Autodesk Inventor part; units mm, degrees
ref_plane "YZ Plane" through (0, 0, 0) normal (1, 0, 0) x (0, 1, 0)
ref_plane "XZ Plane" through (0, 0, 0) normal (0, 1, 0) x (-1, 0, 0)
ref_plane "XY Plane" through (0, 0, 0) normal (0, 0, 1) x (1, 0, 0)
sketch "Sketch3" plane through (0, 0, 0) normal (0, 0, 1) x (1, 0, 0)
  line L0 (-80.5781, 0.8246) -> (-80.5781, 20.7988) construction
  circle A0 centre (-80.5781, 0.8246) radius 13.481
  line L1 (-53.7179, 12.5571) -> (-53.7179, -10.9927)
  arc A1 (-53.7179, -10.9927) -> (-51.5054, -12.9814) centre (-51.7179, -10.9927) ccw
  arc A2 (-51.5054, 14.5458) -> (-53.7179, 12.5571) centre (-51.7179, 12.5571) ccw
  line L2 (36.2229, -3.6088) -> (-51.5054, -12.9814)
  line L3 (38.0104, 3.1845) -> (38.0104, -1.6201)
  line L4 (-80.5781, 0.8246) -> (49.5525, 0.8246) construction
  circle A3 centre (49.6953, -3.8247) radius 5.6609
  line L5 (59.6953, 14.884) -> (59.6953, -12.7998) construction
  spline S0 degree 4 poles (77.9414, 11.0338) (75.5683, 12.9654) (71.7145, 13.0272) (66.8099, 13.9036) (60.7685, 14.7338) (56.2959, 15.3578) (51.7728, 15.9509) (47.2242, 16.5426) (42.6244, 17.1111) (37.9974, 17.6651) (33.3378, 18.1987) (28.6546, 18.7114) (23.9504, 19.2026) (19.2309, 19.6699) (14.5002, 20.1135) (9.7632, 20.5291) (5.025, 20.9191) (0.2903, 21.2792) (-4.4372, 21.6095) (-9.151, 21.9092) (-13.8524, 22.1766) (-18.5268, 22.4102) (-23.2002, 22.6105) (-27.8558, 22.7627) (-32.4748, 22.8704) (-37.0553, 22.9312) (-41.5904, 22.9454) (-46.0738, 22.9127) (-50.5027, 22.8323) (-54.8678, 22.7052) (-59.1755, 22.5324) (-63.394, 22.3084) (-67.5752, 22.0492) (-71.5451, 21.7209) (-75.7777, 21.4072) (-79.04, 20.9063) (-83.4863, 20.5541) (-87.0067, 20.037) (-90.7113, 19.5168) (-94.2172, 18.9459) (-97.6363, 18.3426) (-100.9342, 17.7015) (-104.1216, 17.0263) (-107.1909, 16.3187) (-110.1396, 15.5797) (-112.9656, 14.8117) (-115.6652, 14.0172) (-118.2357, 13.1965) (-120.6759, 12.3541) (-122.9817, 11.4895) (-125.1529, 10.6071) (-127.1857, 9.7065) (-129.0794, 8.7914) (-130.8324, 7.8633) (-132.4429, 6.923) (-133.9096, 5.9737) (-135.2322, 5.016) (-136.4083, 4.0508) (-137.4392, 3.0816) (-138.3215, 2.1025) (-139.0592, 1.1321) (-139.6407, 0.1249) (-140.106, -0.8362) (-140.3589, -2.0477) (-140.602, -2.598) (-140.1166, -5.4607) (-140.0539, -5.4622) (-139.4639, -6.7645) (-138.8842, -7.4979) (-138.1173, -8.3934) (-137.2199, -9.1877) (-136.1721, -9.9852) (-134.9893, -10.738) (-133.6669, -11.4655) (-132.2091, -12.1599) (-130.6156, -12.8245) (-128.8897, -13.4579) (-127.0312, -14.0591) (-125.0439, -14.6296) (-122.9287, -15.1678) (-120.6879, -15.6738) (-118.3241, -16.1476) (-115.8396, -16.5892) (-113.2366, -16.9984) (-110.5176, -17.3742) (-107.6861, -17.7183) (-104.7439, -18.0297) (-101.6943, -18.3095) (-98.5398, -18.5568) (-95.2843, -18.7732) (-91.9297, -18.9579) (-88.48, -19.1131) (-84.9381, -19.2376) (-81.3071, -19.3341) (-77.5906, -19.4015) (-73.7915, -19.4421) (-69.9139, -19.4561) (-65.961, -19.445) (-61.9362, -19.4102) (-57.8434, -19.3518) (-53.6861, -19.2727) (-49.4679, -19.1731) (-45.1932, -19.0538) (-40.8649, -18.9183) (-36.4879, -18.766) (-32.0649, -18.5992) (-27.598, -18.4192) (-23.0941, -18.227) (-18.5434, -18.0273) (-13.9382, -17.8076) (-9.3141, -17.5719) (-4.666, -17.3195) (-0.0002, -17.052) (4.6675, -16.7728) (9.3655, -16.4759) (14.0236, -16.1832) (19.545, -15.7815) (23.3079, -15.6072) (27.1098, -15.1781) (28.8959, -15.0599) knots 0 0 0 0 0 0.024672 0.034555 0.0445 0.054495 0.064543 0.074632 0.084755 0.094911 0.105094 0.115299 0.125521 0.135755 0.145995 0.156237 0.166475 0.176705 0.186921 0.197118 0.207299 0.217463 0.227605 0.23772 0.247796 0.257824 0.267798 0.277713 0.287563 0.297345 0.307053 0.31668 0.326224 0.335555 0.344908 0.354162 0.363308 0.372467 0.381393 0.390196 0.398872 0.407415 0.41582 0.424082 0.432193 0.44015 0.447945 0.455574 0.46303 0.470307 0.477401 0.484305 0.491015 0.497525 0.503831 0.509931 0.515822 0.521506 0.526986 0.53227 0.537373 0.542316 0.547131 0.552525 0.557529 0.562533 0.567581 0.57205 0.576988 0.582082 0.587354 0.592817 0.598478 0.604341 0.610406 0.616671 0.623133 0.629789 0.636632 0.643658 0.650861 0.658236 0.665777 0.673478 0.681333 0.689338 0.697486 0.705771 0.71419 0.722736 0.731403 0.740188 0.749084 0.758087 0.767192 0.776393 0.785687 0.795067 0.804529 0.814069 0.823682 0.833362 0.843106 0.852907 0.862763 0.872667 0.88262 0.892624 0.902675 0.912766 0.92289 0.933033 0.943191 0.953358 0.963531 0.973703 0.984092 1 1 1 1 1
  line L6 (7.5013, -16.4763) -> (50.2906, -13.6435) construction
  arc A4 (44.8353, -17.2546) -> (13.385, -19.3367) centre (31.5327, -54.8885) ccw construction
  line L7 (159.6953, -3.8066) -> (59.6953, -3.8066) construction
  line L8 (-51.5054, 14.5458) -> (36.2229, 5.1732)
  arc A5 (36.2229, -3.6088) -> (38.0104, -1.6201) centre (36.0104, -1.6201) ccw
  arc A6 (38.0104, 3.1845) -> (36.2229, 5.1732) centre (36.0104, 3.1845) ccw
  spline S1 degree 4 poles (78.1029, 11.0141) (76.6463, 11.2227) (73.9909, 10.5042) (70.2765, 8.6041) (66.0429, 5.3938) (62.3889, 1.8499) (60.314, -1.2467) (59.5572, -3.5763) (59.5773, -5.0793) knots 0 0 0 0 0 0.302475 0.43895 0.576633 0.708802 1 1 1 1 1
  spline S2 degree 4 poles (28.8959, -15.0599) (34.0984, -14.7105) (49.269, -14.182) (58.5645, -15.239) (59.5773, -5.0793) knots 0 0 0 0 0 1 1 1 1 1
  line L9 (28.8959, -15.0599) -> (34.0984, -14.7105) construction
  line L10 (34.0984, -14.7105) -> (49.269, -14.182) construction
  line L11 (49.269, -14.182) -> (58.5645, -15.239) construction
  line L12 (58.5645, -15.239) -> (59.5773, -5.0793) construction
  line L13 (-140.4646, -2.8394) -> (159.4818, -3.8173) construction
  line L14 (-132.0856, 0.6333) -> (-132.0856, -6.3667)
  line L15 (-132.0856, -6.3667) -> (-110.3816, -12.3574)
  line L16 (-110.3816, -12.3574) -> (-104.797, -12.3574)
  line L17 (-104.797, -12.3574) -> (-104.797, -18.0156)
  line L18 (-132.0856, 0.6333) -> (-110.3816, 10.553)
  line L19 (-110.3816, 10.553) -> (-104.1736, 10.553)
  line L20 (-104.1736, 10.553) -> (-104.1736, 17.0026)
  line L21 (38.0104, 0.8246) -> (38.0104, -14.6534)
  line L22 (38.0104, 0.8246) -> (38.0104, 17.6585)
  point P0 (0, 0)
  point P1 (17.6589, 23.5628)
  point P2 (75.883, 10.8572)
  point P3 (72.8647, 9.7686)
  point P4 (69.4179, 7.8149)
  point P5 (66.0452, 5.2617)
  point P6 (63.1887, 2.4463)
  point P7 (61.1228, -0.3317)
  point P8 (59.9357, -2.8689)
  point P9 (-160.0931, -3.8671)
  point P10 (28.8959, -15.0599)
  point P11 (69.5533, 13.4647)
  point P12 (65.1899, 14.1023)
  point P13 (60.7936, 14.7318)
  point P14 (56.3207, 15.3468)
  point P15 (51.7945, 15.947)
  point P16 (47.2398, 16.5346)
  point P17 (42.6414, 17.1053)
  point P18 (33.3491, 18.1925)
  point P19 (28.6632, 18.7055)
  point P20 (23.9568, 19.1966)
  point P21 (19.2348, 19.6643)
  point P22 (14.5017, 20.1074)
  point P23 (9.7623, 20.5238)
  point P24 (5.0217, 20.9132)
  point P25 (0.2844, 21.2735)
  point P26 (-4.4451, 21.6038)
  point P27 (-9.1614, 21.9032)
  point P28 (-13.86, 22.1702)
  point P29 (-18.5361, 22.4036)
  point P30 (-23.211, 22.601)
  point P31 (-27.8721, 22.754)
  point P32 (-32.4966, 22.8611)
  point P33 (-37.0797, 22.9217)
  point P34 (-41.6169, 22.9356)
  point P35 (-46.1028, 22.9023)
  point P36 (-50.5329, 22.8216)
  point P37 (-54.9021, 22.6941)
  point P38 (-59.2065, 22.5195)
  point P39 (-63.4406, 22.2977)
  point P40 (-67.6008, 22.0302)
  point P41 (-71.6806, 21.7165)
  point P42 (-75.6814, 21.3591)
  point P43 (-79.1834, 20.9458)
  point P44 (-83.4048, 20.5095)
  point P45 (-87.1309, 20.023)
  point P46 (-90.7527, 19.494)
  point P47 (-94.2725, 18.9266)
  point P48 (-97.6845, 18.3211)
  point P49 (-100.9861, 17.6791)
  point P50 (-107.2438, 16.2934)
  point P51 (-110.1931, 15.553)
  point P52 (-113.0194, 14.7835)
  point P53 (-115.7191, 13.987)
  point P54 (-118.2898, 13.165)
  point P55 (-120.7294, 12.3201)
  point P56 (-123.0349, 11.454)
  point P57 (-125.2048, 10.569)
  point P58 (-127.2364, 9.6666)
  point P59 (-129.1282, 8.7491)
  point P60 (-130.8786, 7.8185)
  point P61 (-132.486, 6.8762)
  point P62 (-133.9488, 5.9245)
  point P63 (-135.2661, 4.9648)
  point P64 (-136.4363, 3.9987)
  point P65 (-137.4592, 3.0275)
  point P66 (-138.3336, 2.0531)
  point P67 (-139.0591, 1.0763)
  point P68 (-139.6352, 0.0983)
  point P69 (-140.0613, -0.8802)
  point P70 (-140.338, -1.8576)
  point P71 (-140.1239, -5.2398)
  point P72 (-139.9547, -5.7022)
  point P73 (-139.492, -6.6066)
  point P74 (-138.8844, -7.4823)
  point P75 (-138.1328, -8.3292)
  point P76 (-137.2384, -9.147)
  point P77 (-136.202, -9.9355)
  point P78 (-135.0249, -10.6943)
  point P79 (-133.7085, -11.4228)
  point P80 (-132.2548, -12.1206)
  point P81 (-130.6648, -12.7879)
  point P82 (-128.941, -13.4239)
  point P83 (-127.0846, -14.0282)
  point P84 (-125.0983, -14.6009)
  point P85 (-122.9839, -15.1415)
  point P86 (-120.7435, -15.6497)
  point P87 (-118.3798, -16.1256)
  point P88 (-115.8952, -16.569)
  point P89 (-113.2918, -16.9797)
  point P90 (-110.5723, -17.3574)
  point P91 (-107.74, -17.7027)
  point P92 (-101.7463, -18.2964)
  point P93 (-98.5909, -18.5451)
  point P94 (-95.3341, -18.7623)
  point P95 (-91.9783, -18.9484)
  point P96 (-88.5271, -19.1041)
  point P97 (-84.9838, -19.2298)
  point P98 (-81.3514, -19.3267)
  point P99 (-77.6332, -19.3951)
  point P100 (-73.8324, -19.4362)
  point P101 (-69.9531, -19.4509)
  point P102 (-65.9985, -19.4404)
  point P103 (-61.9719, -19.4059)
  point P104 (-57.8772, -19.3483)
  point P105 (-53.718, -19.2694)
  point P106 (-49.4979, -19.1701)
  point P107 (-45.2211, -19.0516)
  point P108 (-40.8909, -18.916)
  point P109 (-36.5118, -18.7642)
  point P110 (-32.0871, -18.5977)
  point P111 (-27.6213, -18.418)
  point P112 (-23.1183, -18.2269)
  point P113 (-18.5646, -18.0247)
  point P114 (-13.9566, -17.8054)
  point P115 (-9.3252, -17.5693)
  point P116 (-4.674, -17.317)
  point P117 (-0.0078, -17.05)
  point P118 (4.6686, -16.7695)
  point P119 (9.3513, -16.477)
  point P120 (14.0352, -16.1731)
  point P121 (18.7161, -15.8596)
  point P122 (23.3889, -15.5371)
  point P123 (78.0825, 12.164)
  point P124 (159.2574, -3.8401)
  point P125 (158.8836, -3.8779)
  point P126 (158.3607, -3.9307)
  point P127 (157.6896, -3.9985)
  point P128 (156.8706, -4.081)
  point P129 (155.9046, -4.1779)
  point P130 (154.7931, -4.2892)
  point P131 (153.5367, -4.4143)
  point P132 (152.1372, -4.5532)
  point P133 (150.5955, -4.7056)
  point P134 (148.914, -4.8712)
  point P135 (147.0936, -5.0494)
  point P136 (145.137, -5.2399)
  point P137 (143.0457, -5.4421)
  point P138 (140.8221, -5.6563)
  point P139 (138.4686, -5.8813)
  point P140 (135.9876, -6.1174)
  point P141 (133.3815, -6.3634)
  point P142 (130.6533, -6.6196)
  point P143 (127.8054, -6.8851)
  point P144 (124.8414, -7.1596)
  point P145 (121.7634, -7.4428)
  point P146 (118.5756, -7.7341)
  point P147 (115.2804, -8.0332)
  point P148 (111.8817, -8.3395)
  point P149 (108.3828, -8.6527)
  point P150 (104.787, -8.9722)
  point P151 (101.0985, -9.2974)
  point P152 (97.3206, -9.6283)
  point P153 (93.4572, -9.9643)
  point P154 (89.5122, -10.3048)
  point P155 (85.4898, -10.6492)
  point P156 (81.3936, -10.9969)
  point P157 (77.2284, -11.3479)
  point P158 (72.9975, -11.701)
  point P159 (68.7057, -12.0556)
  point P160 (64.3572, -12.4117)
  point P161 (59.9559, -12.7678)
  point P162 (55.5069, -13.1239)
  point P163 (51.0138, -13.4788)
  point P164 (46.4817, -13.8316)
  point P165 (41.9148, -14.182)
  point P166 (35.7035, -14.3277)
  point P167 (32.6946, -14.8708)
  point P168 (82.2459, 11.5043)
  point P169 (86.3364, 10.8401)
  point P170 (90.3495, 10.1732)
  point P171 (94.2816, 9.5051)
  point P172 (98.1288, 8.837)
  point P173 (101.8872, 8.171)
  point P174 (105.5538, 7.5086)
  point P175 (109.1244, 6.8507)
  point P176 (112.596, 6.1997)
  point P177 (115.9653, 5.5565)
  point P178 (119.2287, 4.9229)
  point P179 (122.3835, 4.3007)
  point P180 (125.4264, 3.6911)
  point P181 (128.3547, 3.0956)
  point P182 (131.1654, 2.5157)
  point P183 (133.8561, 1.9532)
  point P184 (136.4244, 1.4093)
  point P185 (138.8676, 0.8855)
  point P186 (141.1833, 0.383)
  point P187 (143.3697, -0.0964)
  point P188 (145.4247, -0.5518)
  point P189 (147.3462, -0.9817)
  point P190 (149.1327, -1.3852)
  point P191 (150.7821, -1.7608)
  point P192 (152.2935, -2.1073)
  point P193 (153.6651, -2.4241)
  point P194 (154.8954, -2.7103)
  point P195 (155.9838, -2.9647)
  point P196 (156.9291, -3.187)
  point P197 (157.7307, -3.376)
  point P198 (158.3871, -3.5317)
  point P199 (158.8986, -3.6529)
  dimension "d3" = 26.962
  dimension "d6" = 11.3219
  dimension "d7" = 110
  dimension "d8" = 100
  dimension "d9" = 2
  dimension "d11" = 4.6493
  dimension "d25" = 7
  dimension "d26" = 3.5
  dimension "d27" = 8.379
  dimension "d28" = 30.083
  dimension "d29" = 5
  dimension "d30" = 5
  dimension "d31" = 59.8865
extrude "Extrusion3" add sketch "Sketch3" along normal blind 90.75 contours L22 S0 S1 S2 L21 L3
sketch "Sketch4" plane through (0, 0, 90.75) normal (0, 0, 1) x (1, 0, 0)
  circle A0 centre (49.6953, -3.8247) radius 5.6609
  line L0 (44.0343, -3.8247) -> (38.0104, -3.8247) construction
  line L1 (38.0104, 17.6585) -> (38.0104, -14.6534)
  line L2 (44.5647, -2.8247) -> (37.4801, -2.8247)
  line L3 (37.4801, -2.8247) -> (37.4801, -4.8247)
  line L4 (37.4801, -4.8247) -> (44.5647, -4.8247)
  line L5 (44.5647, -4.8247) -> (44.5647, -2.8247)
  line L6 (44.5647, -2.8247) -> (37.4801, -4.8247) construction
  line L7 (37.4801, -2.8247) -> (44.5647, -4.8247) construction
  point P0 (0, 0)
  point P1 (41.0224, -3.8247)
  dimension "d34" = 2
extrude "Extrusion4" cut sketch "Sketch4" against normal blind 154.75 contours L2 L5 L4 A0 | A0 L4 L1 L2 | L1 L4 L3 L2 picked at (44.3912, -3.9363)
properties part number "4P.01.01.11-TW-v1-WingRibWFlapSingle" material "Polyurethane Foam"
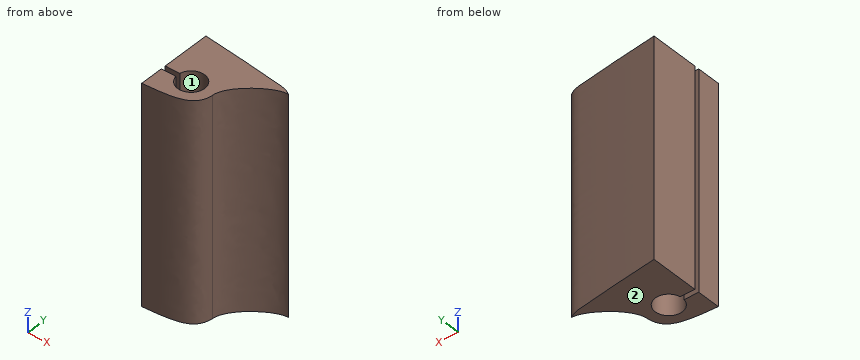
For this review, take the finished solid that the model builds, in its own axes (mm). Face numbers are marked on the shaded views. Give positions to 0.01 mm unless a question says otherwise; leave off trailing zeros. Answer in a Markdown table with one row per item. Add a question column.
(1) Wall thickness on probe 1 along Y at (x, z) = (45.5, 46.5); probe 2 along Y at (x, z) = (47.5, 39); probe 3 along X at (y, z) = (0, 8.5): over which ranges is each line inside the solid? List them lowest first. Write a range as [from, to].
(2) Mouldability with a two-part tool opening along Y and no side actions: class the marked faces 1 and 2 as +Y half, -Y half, draft (parallel to the pull), parting line (faces both ways), or undercut.
(3) For pin 1 (5 mm diameter, centred on y = 3, z = 67, fed in from +X); pin 2 (12 mm diameter, centred on x = 55, z = 12.5, fed in from +Y); pin 3 (14.5 mm diameter, centred on x = 49.7, y = -3.82, fed in from +Z); pin 4 (10 mm diameter, centred on x = 51, z = 14, fed in from +Y), all flat-tipped, find the tip position at first contact; note any pin that passes through.
Evaluation:
| question | item | result |
|---|---|---|
| 1 | probe 1 | y = [-14.23, -7.63], [-0.02, 16.75] |
| 1 | probe 2 | y = [-14.03, -9.04], [1.39, 16.5] |
| 1 | probe 3 | x = [38.01, 45.52], [53.87, 61.33] |
| 2 | face 1 | undercut |
| 2 | face 2 | draft |
| 3 | pin 1 | stops at x = 66.32 |
| 3 | pin 2 | stops at y = 16.31 |
| 3 | pin 3 | stops at z = 90.75 |
| 3 | pin 4 | stops at y = 16.69 |
